```python
from build123d import *

# Parameters (mm, degrees)
SKETCH1_R           = 12
SKETCH1_R_2         = 10
BOSS_EXTRUDE1_DEPTH = 5


with BuildPart() as part:
    # Sketch1 → Boss-Extrude1 (new body)
    # profile 1 of 2: a face of its own
    with BuildSketch(Plane.XY):
        with BuildLine():
            Line((-12, -12), (-12, 0))
            ThreePointArc((-12, 0), (0, 12), (12, 0))
            Line((12, 0), (12, -12))
            Line((12, -12), (23.395271001, -12))
            Line((23.395271001, -12), (23.395271001, -10))
            Line((23.395271001, -10), (14, -10))
            Line((14, -10), (14, 0))
            ThreePointArc((14, 0), (0, 14), (-14, 0))
            Line((-14, 0), (-14, -10))
            Line((-14, -10), (-23.395271001, -10))
            Line((-23.395271001, -10), (-23.395271001, -12))
            Line((-23.395271001, -12), (-12, -12))
        make_face()
    # profile 2 of 2: a face of its own
    with BuildSketch(Plane.XY):
        Circle(SKETCH1_R)
        Circle(SKETCH1_R_2, mode=Mode.SUBTRACT)
    extrude(amount=BOSS_EXTRUDE1_DEPTH)


solid = part.part
```
The listing builds one solid part. Answer for the finished solid, in the listing's coordinates (mm). A direction names the side the tool comes from. Give positions to 0.01 mm unless a question says otherwise; leave off trailing zeros. Order: outer loops, then holes, each group sorted by start corner. A loop starts at its lowest first (then second) coordinate and runs counter-clockwise, first axis right, second up. Notation, with made-up numbers: (-17, 7.5) -> (34, 7.5) arc R17 ccw to (34, 21.5) -> close; hole circle Ø8 at (31, -2). An arc over 180 degrees is marked (long way). Answer as CSV lines item,"result". Start each with the question number.
Q1. Given pin 1 (1.5 mm diameter, centred on y = -7.5, z = 2, fed in from -X); pin 2 (1.5 mm diameter, centred on x = 5, z = 1.5, fed in from +Y); pin 3 (1.5 mm diameter, centred on x = -21, z = 3.5, fed in from +Y), each flat-ended and moving along its own axis, determine where each tip first touches the part or whether it passes through.
Q2. Which of the six approach directions +Z, -Z, +X, -X, +Y, -Y give full straight-line access (tool end or side, diameter ignored) to faces 1 (the flat face through (-19, -10, 2)), 2 (the flat face through (19, -10, 2)), 3 (the flat face through (-23.395, -11, 2))?
Q3. Find the intervals of material crossed by L1, parallel to X at y = -8.5, z = 2.8; L2, parallel to Y at x = 0, z = 3; L3, parallel to Y at x = -5, z = 4.7, in increasing order.
Q4. A cutting plane is placed at A-A (x = 0). Determine the outline of the cut face in (y, z), then the cut area to 3 significant figures.
Q5. Determine the mould class of faces 4 (the cylindrical face through (0, -12, 2)), 5 (the flat face through (12, -6, 2)), 6 (the flat face through (-14, -5, 2)), 7 (the flat face through (3, -10, 0)) for opening direction X: pulls with the +X half, pulls with the -X half, needs draft (parallel to the pull), parting line crosses it, or undercut.
Q6. A cutting plane is placed at D-D (y = 6.25). Determine the outline of the cut face in (x, z), then the cut area to 3 significant figures.
Q7. A cutting plane is placed at B-B (z = 2.25). Determine the outline of the cut face in (x, y), then the cut area to 3 significant figures.
Q8. A cutting plane is placed at C-C (y = -9.5). Determine the outline of the cut face in (x, z).
Results found:
1,pin 1,"x = -14"
1,pin 2,"y = 13.34"
1,pin 3,"y = -10"
2,face 1,"+Z, -Z, -X, +Y"
2,face 2,"+Z, -Z, +X, +Y"
2,face 3,"+Z, -Z, -X, +Y, -Y"
3,L1,"-14 to -12, -8.47 to -5.27, 5.27 to 8.47, 12 to 14"
3,L2,"-12 to -10, 10 to 14"
3,L3,"-10.91 to -8.66, 8.66 to 13.08"
4,outline,"(-12, 0) -> (-10, 0) -> (-10, 5) -> (-12, 5) -> close; (10, 0) -> (14, 0) -> (14, 5) -> (10, 5) -> close"
4,area,"30.0 mm2"
5,face 4,"undercut"
5,face 5,"undercut"
5,face 6,"pulls with the -X half"
5,face 7,"needs draft"
6,outline,"(-12.53, 0) -> (-7.81, 0) -> (-7.81, 5) -> (-12.53, 5) -> close; (7.81, 0) -> (12.53, 0) -> (12.53, 5) -> (7.81, 5) -> close"
6,area,"47.2 mm2"
7,outline,"(-23.4, -12) -> (-12, -12) -> (-12, 0) arc R12 ccw to (12, 0) -> (12, -12) -> (23.4, -12) -> (23.4, -10) -> (14, -10) -> (14, 0) arc R14 ccw to (-14, 0) -> (-14, -10) -> (-23.4, -10) -> close; hole circle Ø20 at (0, 0)"
7,area,"305 mm2"
8,outline,"(-14, 0) -> (-12, 0) -> (-12, 5) -> (-14, 5) -> close; (-7.33, 0) -> (-3.12, 0) -> (-3.12, 5) -> (-7.33, 5) -> close; (3.12, 0) -> (7.33, 0) -> (7.33, 5) -> (3.12, 5) -> close; (12, 0) -> (14, 0) -> (14, 5) -> (12, 5) -> close"
